Build history of the part. All positions in model axes, mm. Face numbers are marked on the shaded views. A direction names the side the tool comes from. Round coordinates to 2 decimals unless told otherwise and drop trailing zeros. Loops run counter-clockwise (first coordinate to the right, second up) from the corner with the lowest first, then second, coordinate; pieces in that order, holes last. Notation, with made-up numbers: (-33, 15) -> (-21, 15) arc R29 ccw to (-21, 42) -> close; hole circle Ø5 at (38.5, 48.25). An arc over 180 degrees is marked (long way). Put each result on its own line as item: value. Start each with the question number.
Item 1: Flat gauge pins, fed straight in: pin 1 Ø3 at (x, y) = (-7, 15.5) entering from -Z; pin 2 Ø4.5 at (y, z) = (15.83, 49.18) entering from +X; pin 3 Ø12 at (x, y) = (-12.5, -18.5) entering from -Z. Where does each tip first touch, or does it go through?
Item 2: Tool access for the marked faces 1, 2 and 3: list every direction of +Z, -Z, +X, -X, +Y, -Y with a clear straight run to the whole face (end or side of a thin tool).
Item 3: Cut at B-B, the plane x = 8. Count the separate pieces of the cut face and the enclosed holes in it, plus the area to 3 significant figures.
Item 4: Cut at A-A, the plane y = 0. List the corners of the cut face in (x, z), plus the area to 3 significant figures.
Item 5: Drill centre lines: probe 1 along X at (y, z) = (15.5, 42.2); probe 2 along Y at (x, z) = (-15, 70.5); probe 3 along X at (y, z) = (0, 83.5). Where is each one in solid material? Low to high. Write a range as [from, to].
Item 6: Pull direction X, two halves, no side cores. Call the marked faces 4, 5 and 6: +X half, -X half, draft (parallel to the pull), parting line (faces both ways), or undercut.
```python
from build123d import *

# Parameters (mm, degrees)
SKETCH029_W     = 42.3
SKETCH029_H     = 87
PAD013_DEPTH    = 4
SKETCH030_W     = 42.3
SKETCH030_H     = 4
SKETCH030_H_2   = 14
PAD014_DEPTH    = 42.3
SKETCH032_R     = 11
POCKET013_DEPTH = 14
SKETCH031_R     = 1.7
SKETCH031_R_2   = 12
POCKET014_DEPTH = 5
SKETCH033_W     = 87
SKETCH033_H     = 46.3
PAD015_DEPTH    = 4
SKETCH034_W     = 87
SKETCH034_H     = 46.3
PAD016_DEPTH    = 4
SKETCH035_R     = 2
POCKET015_DEPTH = 14
POCKET016_DEPTH = 51
SKETCH037_R     = 12.795503
POCKET017_DEPTH = 51
SKETCH038_R     = 2
POCKET018_DEPTH = 5
FILLET002_R     = 1


with BuildPart() as part:
    # Sketch029 → Pad013 (new body)
    with BuildSketch(Plane.YZ):
        with Locations((0, 43.5)):
            Rectangle(SKETCH029_W, SKETCH029_H)
    extrude(amount=PAD013_DEPTH)

    # Sketch030 (on Face6 of Pad013) → Pad014 (join)
    with BuildSketch(Plane.YZ.offset(4)):
        with Locations((0, 42.178345)):
            Rectangle(SKETCH030_W, SKETCH030_H)
        with Locations((0, 80)):
            Rectangle(SKETCH030_W, SKETCH030_H_2)
    extrude(amount=PAD014_DEPTH)

    # Sketch032 (on Face13 of Pad014) → Pocket013 (cut)
    with BuildSketch(Plane(origin=(0, 0, 87), x_dir=(0, -1, 0), z_dir=(0, 0, 1))):
        with Locations((0, 25)):
            Circle(SKETCH032_R)
    extrude(amount=-POCKET013_DEPTH, mode=Mode.SUBTRACT)

    # Sketch031 (on Face12 of Pad014) → Pocket014 (cut)
    with BuildSketch(Plane.YX.offset(-40.178345)):
        with Locations((-15.5, 40.65)):
            Circle(SKETCH031_R)
        with Locations((15.5, 40.65)):
            Circle(SKETCH031_R)
        with Locations((15.5, 9.65)):
            Circle(SKETCH031_R)
        with Locations((-15.5, 9.65)):
            Circle(SKETCH031_R)
        with Locations((0, 25)):
            Circle(SKETCH031_R_2)
    extrude(amount=-POCKET014_DEPTH, mode=Mode.SUBTRACT)

    # Sketch033 (on Face3 of Pocket014) → Pad015 (join)
    with BuildSketch(Plane.ZX.offset(21.15)):
        with Locations((43.5, 23.15)):
            Rectangle(SKETCH033_W, SKETCH033_H)
    extrude(amount=PAD015_DEPTH)

    # Sketch034 (on Face2 of Pad015) → Pad016 (join)
    with BuildSketch(Plane(origin=(0, -21.15, 0), x_dir=(0, 0, -1), z_dir=(0, -1, 0))):
        with Locations((-43.5, 23.15)):
            Rectangle(SKETCH034_W, SKETCH034_H)
    extrude(amount=PAD016_DEPTH)

    # Sketch035 (on Face22 of Pad016) → Pocket015 (cut)
    with BuildSketch(Plane(origin=(0, 0, 87), x_dir=(0, -1, 0), z_dir=(0, 0, 1))):
        with Locations((-15.5, 40.65)):
            Circle(SKETCH035_R)
        with Locations((15.5, 40.65)):
            Circle(SKETCH035_R)
        with Locations((15.5, 9.65)):
            Circle(SKETCH035_R)
        with Locations((-15.5, 9.65)):
            Circle(SKETCH035_R)
    extrude(amount=-POCKET015_DEPTH, mode=Mode.SUBTRACT)

    # Sketch036 (on Face13 of Pocket015) → Pocket016 (cut)
    with BuildSketch(Plane.ZX.offset(25.15)):
        Polygon((0, 4), (40, 46.3), (0, 46.3), align=None)
    extrude(amount=-POCKET016_DEPTH, mode=Mode.SUBTRACT)

    # Sketch037 (on Face7 of Pocket016) → Pocket017 (cut)
    with BuildSketch(Plane(origin=(0, -25.15, 0), x_dir=(0, 0, -1), z_dir=(0, -1, 0))):
        with Locations((-60.230976, 25.198834)):
            Circle(SKETCH037_R)
    extrude(amount=-POCKET017_DEPTH, mode=Mode.SUBTRACT)

    # Sketch038 → Pocket018 (cut)
    with BuildSketch(Plane.YZ.offset(4)):
        with Locations((-15.828298, 68.323807)):
            Circle(SKETCH038_R)
        with Locations((15.828298, 68.323807)):
            Circle(SKETCH038_R)
        with Locations((-15.828298, 49.17934)):
            Circle(SKETCH038_R)
        with Locations((15.828298, 49.17934)):
            Circle(SKETCH038_R)
    extrude(amount=-POCKET018_DEPTH, mode=Mode.SUBTRACT)

    # Fillet002
    fillet002_edges = [part.edges().sort_by_distance(p)[0] for p in [
        (2, -25.15, 0),
        (25.15, -25.15, 20),
        (0, -25.15, 43.5),
        (46.3, -25.15, 63.5),
        (23.15, -25.15, 87),
        (25.198834, -25.15, 73.026479),
        (2, 25.15, 0),
        (25.15, 25.15, 20),
        (0, 25.15, 43.5),
        (46.3, 25.15, 63.5),
        (23.15, 25.15, 87),
        (25.198834, 25.15, 73.026479),
    ]]
    fillet(fillet002_edges, radius=FILLET002_R)


with BuildPart() as part_1:
    # Body013 placement: moved
    add(part.part.moved(Location((-25, 0, 0))))


solid = part_1.part
```
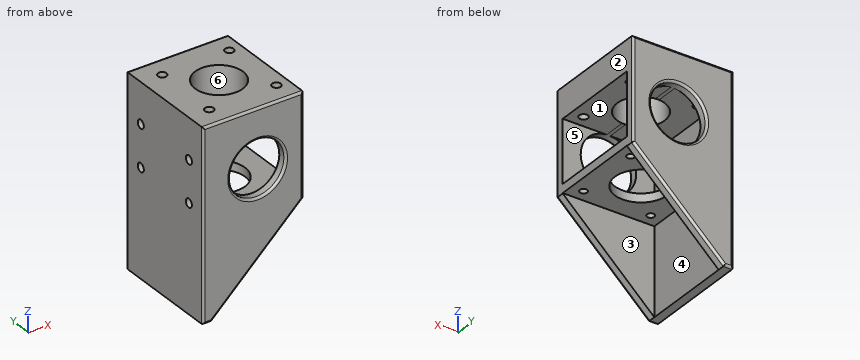
Reply:
1. pin 1: stops at z = 40.18
1. pin 2: stops at x = -21
1. pin 3: stops at z = 2.95
2. face 1: +X
2. face 2: +Z, -Z, +X, +Y, -Y
2. face 3: -Z, +X
3. separate pieces: 4
3. enclosed holes: 0
3. area: 791 mm^2
4. outline: (-25, 0) -> (-21, 0) -> (-21, 40.18) -> (-12, 40.18) -> (-12, 44.18) -> (-21, 44.18) -> (-21, 73) -> (-11, 73) -> (-11, 87) -> (-25, 87) -> close; (11, 73) -> (21.3, 73) -> (21.3, 87) -> (11, 87) -> close; (12, 40.18) -> (21.3, 40.18) -> (21.3, 44.18) -> (12, 44.18) -> close
4. area: 705 mm^2
5. probe 1: x = [-25, -17.05], [-13.65, 13.95], [17.35, 21.3]
5. probe 2: y = [-25.15, -21.15], [21.15, 25.15]
5. probe 3: x = [-25, -11], [11, 21.3]
6. face 4: +X half
6. face 5: draft
6. face 6: undercut
